Part model, mm, in its own coordinate system. Round coordinates to 2 decimals unless told otherwise and drop trailing zeros. Loops run counter-clockwise (first coordinate to the right, second up) from the corner with the lowest first, then second, coordinate; pieces in that order, holes last.
1) Probe line 1 (X direction, y = -1.2, z = 36.5); line 2 (X direction, y = -2.4, z = -5); line 3 (Z direction, x = 37, y = -1.1). List the from-to ranges inside material, lowest first.
2) Band-saw the part on A-A, the plane z = 38.5. Write the cut outline in (x, y) (3 decimals).
3) Band-saw the part on B-B, the plane y = -1.55. Write the cut outline in (x, z) (3 decimals).
4) Drop flat-ended pins along their axis: P1, Ø1.6, axis at y = -1, z = -41, coming from the +X side; P2, Ø1.6, axis at x = 94.5, y = -2, coming from the -Z side; P3, Ø1.6, axis at x = 49, y = -1, coming from the +Z side. Give the stop position or say it passes through.
5) Band-saw the part on C-C, the plane x = 44. Write the cut outline in (y, z) (3 decimals), then the cut area to 3 significant figures.
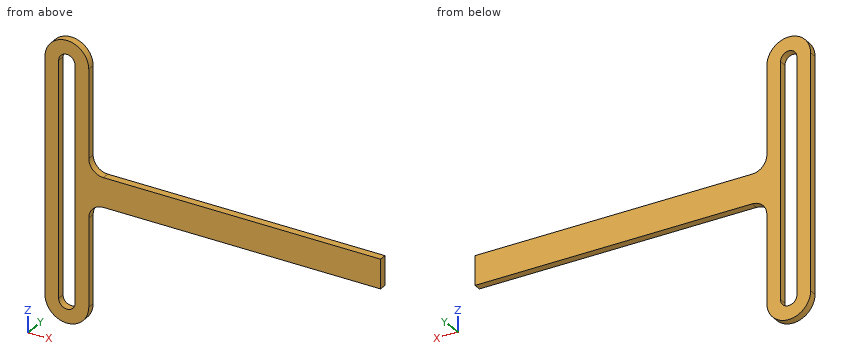
from build123d import *

# Parameters (mm, degrees)
F1_DEPTH = 3.175
F3_DEPTH = 25.4


with BuildPart() as f1:
    # F0 (on Front) → F1 (new body)
    with BuildSketch(Plane.XZ):
        with BuildLine():
            Line((127, 0), (6.35, 0))
            ThreePointArc((6.35, 0), (1.859872, 1.859872), (0, 6.35))
            Line((0, 6.35), (0, 44.45))
            ThreePointArc((0, 44.45), (-9.525, 53.975), (-19.05, 44.45))
            Line((-19.05, 44.45), (-19.05, -57.15))
            ThreePointArc((-19.05, -57.15), (-9.525, -66.675), (0, -57.15))
            Line((0, -57.15), (0, -19.05))
            ThreePointArc((0, -19.05), (1.859872, -14.559872), (6.35, -12.7))
            Line((6.35, -12.7), (127, -12.7))
            Line((127, -12.7), (127, 0))
        make_face()
    extrude(amount=F1_DEPTH)

    # F2 (on face) → F3 (cut)
    with BuildSketch(Plane.XZ.offset(3.175)):
        with BuildLine():
            Line((-5.969, 6.35), (-5.969, 44.45))
            ThreePointArc((-5.969, 44.45), (-9.525, 48.006), (-13.081, 44.45))
            Line((-13.081, 44.45), (-13.081, -57.15))
            ThreePointArc((-13.081, -57.15), (-9.525, -60.706), (-5.969, -57.15))
            Line((-5.969, -57.15), (-5.969, -19.05))
            Line((-5.969, -19.05), (-5.969, 6.35))
        make_face()
    extrude(amount=-F3_DEPTH, mode=Mode.SUBTRACT)


solid = f1.part
Reported:
1. line 1: x = -19.05 to -13.08, -5.97 to 0
1. line 2: x = -19.05 to -13.08, -5.97 to 127
1. line 3: z = -12.7 to 0
2. outline: (-19.05, -3.175) - (-13.081, -3.175) - (-13.081, 0) - (-19.05, 0) - close; (-5.969, -3.175) - (0, -3.175) - (0, 0) - (-5.969, 0) - close
3. outline: (-19.05, -57.15) arc R9.525 ccw to (0, -57.15) - (0, -19.05) arc R6.35 cw to (6.35, -12.7) - (127, -12.7) - (127, 0) - (6.35, 0) arc R6.35 cw to (0, 6.35) - (0, 44.45) arc R9.525 ccw to (-19.05, 44.45) - close; hole (-13.081, -57.15) arc R3.556 ccw to (-5.969, -57.15) - (-5.969, 44.45) arc R3.556 ccw to (-13.081, 44.45) - close
4. P1: stops at x = 0
4. P2: stops at z = -12.7
4. P3: stops at z = 0
5. outline: (-3.175, -12.7) - (0, -12.7) - (0, 0) - (-3.175, 0) - close
5. area: 40.3 mm2
